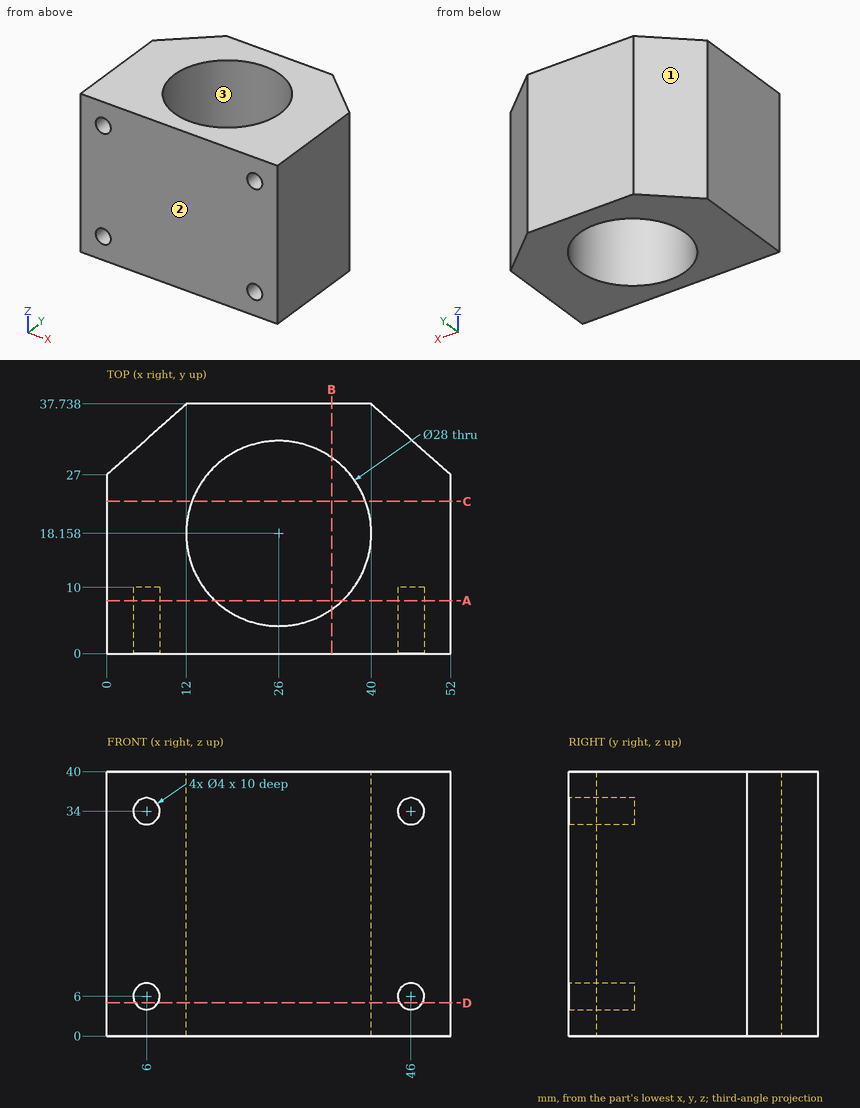
The drawing under review shows one solid part. Ordinate dimensions are in mm from its lowest x, y, z. Round coordinates to 2 decimals unless told otherwise and drop trailing zeros. Write each loop counter-clockwise with the first axis right and the second up, starting at its lowest first coordinate (ties: lowest second). Pieces come first, ordered by that corner, then holes. Notation, with made-up numbers: (67.5, -8.75) - (83.5, -8.75) arc R19 ccw to (83.5, 15.25) - close; hole circle Ø3 at (-22.75, 89). An arc over 180 degrees is marked (long way). Use one line per item in the form item = value.
Q1. Insertion check: pin 1 Ø8 at (x, z) = (7.5, 32.5) entering from +Y; pin 2 Ø3 at (x, z) = (6, 34) entering from +Y; pin 3 Ø1 at (y, z) = (28.5, 16) entering from -X. Each pin has a flat end and moves straight along its axis. Give the tip position at first contact, or say it passes through.
Answer key:
pin_1 = 37.29
pin_2 = 33.71
pin_3 = 1.12
Q2. Consider section A-A (y = 8). State the section outline as (x, z) points, and give its area (3 significant figures).
Answer key:
outline = (0, 0) - (16.37, 0) - (16.37, 40) - (0, 40) - close; (35.63, 0) - (52, 0) - (52, 40) - (35.63, 40) - close; hole circle Ø4 at (6, 6); hole circle Ø4 at (6, 34); hole circle Ø4 at (46, 6); hole circle Ø4 at (46, 34)
area = 1,260 mm2
Q3. Consider section D-D (z = 5). State the section outline as (x, y) points, and give its area (3 significant figures).
Answer key:
outline = (0, 0) - (4.27, 0) - (4.27, 10) - (7.73, 10) - (7.73, 0) - (44.27, 0) - (44.27, 10) - (47.73, 10) - (47.73, 0) - (52, 0) - (52, 27) - (40, 37.74) - (12, 37.74) - (0, 27) - close; hole circle Ø28 at (26, 18.16)
area = 1,150 mm2
Q4. Consider section C-C (y = 23). State the section outline as (x, z) points.
Answer key:
outline = (0, 0) - (12.86, 0) - (12.86, 40) - (0, 40) - close; (39.14, 0) - (52, 0) - (52, 40) - (39.14, 40) - close
Q5. For line 1 (X direction, y = 3, z = 34); line 2 (X direction, y = 7, z = 34) (1 decimal); line 3 (X direction, y = 5.25, z = 6), list the stretches that pass through material, from the lowest coordinate up. Write a range as [from, to].
Answer key:
line_1 = [0, 4], [8, 44], [48, 52]
line_2 = [0, 4], [8, 17.5], [34.5, 44], [48, 52]
line_3 = [0, 4], [8, 20.58], [31.42, 44], [48, 52]
Q6. Draft analysis for pull direction X (two halves, no side actions). For the marked faces 1, 2 and 3, state which applies: +X half, -X half, draft (parallel to the pull), parting line (faces both ways), or undercut.
Answer key:
face_1 = -X half
face_2 = draft
face_3 = undercut
Q7. Consider section B-B (x = 34). State the section outline as (y, z) points, and give its area (3 significant figures).
Answer key:
outline = (0, 0) - (6.67, 0) - (6.67, 40) - (0, 40) - close; (29.65, 0) - (37.74, 0) - (37.74, 40) - (29.65, 40) - close
area = 590 mm2
